Can you work these out from the model? Positions are in its coordinate system, mm. A direction names the side the tool comes from. Coordinates: 2 decimals unless noted, no trailing zeros. Order: outer loops, then holes, each group sorted by start corner. A loop starts at its lowest first (then second) coordinate and runs counter-clockwise, first axis right, second up. Notation, with made-up numbers: M 75.5,79.5 L 133.5,79.5 A17 cw 133.5,95.5 Z; hole C 36,-37 d4. An arc over 180 degrees is marked long. Answer as CSV lines item,"result". Start each with the question number.
1. If we section it at A-A (z = 3.5): List the corners of the cut face in (x, y) for me (3 decimals).
2. If we section it at B-B (x = -1): List the corners of the cut face in (y, z) for me, plus the area to 3 significant figures.
3. If we section it at D-D (x = -9): List the corners of the cut face in (y, z) for me (3 decimals), plus the area to 3 significant figures.
4. Will these pins go through, and if not, where does the flat tip stop? pin 1 (8 mm diameter, centred on x = 2.5, y = -4, fed in from +Z); pin 2 (0.5 mm diameter, centred on x = 15, y = 2, fed in from +Z); pin 3 (1.5 mm diameter, centred on y = -8.5, z = 13.5, fed in from +X); pin 4 (3 mm diameter, centred on x = -22, z = 12, fed in from -Y).
5. If we section it at C-C (y = -6): List the corners of the cut face in (x, z) for me, plus the area to 3 significant figures.
6. I need wall thicknesses on line 1 along X through (y, z) = (3.75, 5); line 2 along Z through (x, y) = (-22, -8.85); line 3 along Y through (x, z) = (19, 2.4). Which ranges of each line are inside material? Lowest first, please. Write a range as from..to.
7. On a 3-axis mill with a long thin cutter (end or side, diameter ignored), from which of +Z, -Z, +X, -X, +Y, -Y can I reach the whole of each face in a straight line? I mean faces 1 (the face through (-17.414, -7.986, 13.368)), 2 (the face through (-16, 4, 4)), 3 (the face through (15.5, 0, 5)). Say none if no direction works.
8. If we mould it in two halves opening along Y, with no side actions, what happens to faces 4 (the face through (-13.6, -9, 13.2)), 5 (the face through (-10.673, 0.074, 2.958)), 6 (the face through (-12.61, -7.99, 13.41))? For each: released by +Y, released by -Y, zero draft, split by the parting line, or undercut.
```python
from build123d import *

# Parameters (mm, degrees)
SKETCH1_W           = 50
SKETCH1_H           = 20
SKETCH1_R           = 3.55
SKETCH1_R_2         = 1.675
SKETCH1_R_3         = 4
SKETCH1_R_4         = 2.4
SKETCH1_W_2         = 8.5
SKETCH1_H_2         = 14
BOSS_EXTRUDE1_DEPTH = 6
SKETCH3_W           = 11
SKETCH3_H           = 20
CUT_EXTRUDE2_DEPTH  = 3
SKETCH4_W           = 12.1
SKETCH4_H           = 20
CUT_EXTRUDE4_DEPTH  = 2
BOSS_EXTRUDE3_START = -3
SKETCH6_W           = 15
SKETCH6_H           = 20
BOSS_EXTRUDE3_DEPTH = 3
SKETCH7_R           = 1.65
CUT_EXTRUDE5_DEPTH  = 3
CUT_EXTRUDE6_DEPTH  = 2
SKETCH10_W          = 7
SKETCH10_H          = 20
SKETCH10_W_2        = 10
CUT_EXTRUDE7_DEPTH  = 3


with BuildPart() as part:
    # Sketch1 → Boss-Extrude1 (new body)
    with BuildSketch(Plane.XY):
        Rectangle(SKETCH1_W, SKETCH1_H)
        with Locations((-17, 0)):
            Circle(SKETCH1_R, mode=Mode.SUBTRACT)
        with Locations((-9, 0)):
            Circle(SKETCH1_R_2, mode=Mode.SUBTRACT)
        with Locations((-1, 0)):
            Circle(SKETCH1_R_3, mode=Mode.SUBTRACT)
        with Locations((19, 0)):
            Circle(SKETCH1_R_4, mode=Mode.SUBTRACT)
        with Locations((9, 0)):
            Rectangle(SKETCH1_W_2, SKETCH1_H_2, mode=Mode.SUBTRACT)
    extrude(amount=BOSS_EXTRUDE1_DEPTH)

    # Sketch3 → Cut-Extrude2 (cut)
    with BuildSketch(Plane.XY.offset(6)):
        with Locations((9, 0)):
            Rectangle(SKETCH3_W, SKETCH3_H)
    extrude(amount=-CUT_EXTRUDE2_DEPTH, mode=Mode.SUBTRACT)

    # Sketch4 → Cut-Extrude4 (cut)
    with BuildSketch(Plane.XY.offset(6)):
        with Locations((-17, 0)):
            Rectangle(SKETCH4_W, SKETCH4_H)
    extrude(amount=-CUT_EXTRUDE4_DEPTH, mode=Mode.SUBTRACT)

    # Sketch6 → Boss-Extrude3 (add)
    with BuildSketch(Plane.XZ.offset(10).offset(BOSS_EXTRUDE3_START)):
        with Locations((-17.5, 10)):
            Rectangle(SKETCH6_W, SKETCH6_H)
    extrude(amount=BOSS_EXTRUDE3_DEPTH)

    # Sketch7 → Cut-Extrude5 (cut)
    with BuildSketch(Plane(origin=(0, -7, 0), x_dir=(1, 0, 0), z_dir=(0, 1, 0))):
        with Locations(Location((-22, -12, 0), (0, 0, 180))):
            Circle(SKETCH7_R)
        with Locations(Location((-15, -12, 0), (0, 0, 180))):
            Circle(SKETCH7_R)
    extrude(amount=-CUT_EXTRUDE5_DEPTH, mode=Mode.SUBTRACT)

    # Sketch8 → Cut-Extrude6 (cut)
    with BuildSketch(Plane(origin=(0, -7, 0), x_dir=(1, 0, 0), z_dir=(0, 1, 0))):
        Polygon((-13.397853003, -9.225), (-16.602146997, -9.225), (-18.204293994, -12), (-16.602146997, -14.775), (-13.397853003, -14.775), (-11.795706006, -12), align=None)
    extrude(amount=-CUT_EXTRUDE6_DEPTH, mode=Mode.SUBTRACT)

    # Sketch10 → Cut-Extrude7 (cut)
    with BuildSketch(Plane.XY.offset(6)):
        with Locations((19, 0)):
            Rectangle(SKETCH10_W, SKETCH10_H)
        with Locations((-1.5, 0)):
            Rectangle(SKETCH10_W_2, SKETCH10_H)
    extrude(amount=-CUT_EXTRUDE7_DEPTH, mode=Mode.SUBTRACT)


solid = part.part
```
Solved:
1,outline,"M -25,-10 L -6.5,-10 L -6.5,10 L -25,10 Z; M 14.5,-10 L 15.5,-10 L 15.5,10 L 14.5,10 Z; M 22.5,-10 L 25,-10 L 25,10 L 22.5,10 Z; hole C -17,0 d7.1; hole C -9,0 d3.35"
2,outline,"M -10,0 L -4,0 L -4,3 L -10,3 Z; M 4,0 L 10,0 L 10,3 L 4,3 Z"
2,area,"36.0 mm²"
3,outline,"M -10,0 L -1.675,0 L -1.675,6 L -10,6 Z; M 1.675,0 L 10,0 L 10,6 L 1.675,6 Z"
3,area,"99.9 mm²"
4,pin 1,"z = 3"
4,pin 2,"z = 6"
4,pin 3,"x = -10"
4,pin 4,"through"
5,outline,"M -25,0 L 4.75,0 L 4.75,3 L -6.5,3 L -6.5,6 L -10.95,6 L -10.95,4 L -23.05,4 L -23.05,6 L -25,6 Z; M 13.25,0 L 25,0 L 25,6 L 22.5,6 L 22.5,3 L 15.5,3 L 15.5,6 L 14.5,6 L 14.5,3 L 13.25,3 Z"
5,area,"166 mm²"
6,line 1,"-25..-23.05, -10.95..-6.5, 14.5..15.5, 22.5..25"
6,line 2,"0..10.35, 13.65..20"
6,line 3,"-10..-2.4, 2.4..10"
7,face 1,"+Y"
7,face 2,"+Z, +Y"
7,face 3,"+Z, +Y, -Y"
8,face 4,"released by +Y"
8,face 5,"undercut"
8,face 6,"zero draft"
